Geometry: final body of the model. Coordinates: model frame, mm. Face numbers are marked on the shaded views. A direction names the side the tool comes from. Round coordinates to 2 decimals unless told otherwise and drop trailing zeros. Order: outer loops, then holes, each group sorted by start corner. A loop starts at its lowest first (then second) coordinate and runs counter-clockwise, first axis right, second up. Notation, with made-up numbers: (38.25, -2.5) -> (89.25, -2.5) arc R33 cw to (89.25, 34.5) -> close; hole circle Ø11 at (-28.5, 5.25). An arc over 180 degrees is marked (long way). Put each result on its own line as item: value.
```python
from build123d import *

# Parameters (mm, degrees)
SKETCH10_R           = 4.05
BOSS_EXTRUDE12_DEPTH = 10
SKETCH11_R           = 35
BOSS_EXTRUDE13_DEPTH = 40.8
SKETCH12_R           = 4
BOSS_EXTRUDE14_DEPTH = 6
SKETCH13_R           = 19.993
BOSS_EXTRUDE15_DEPTH = 75
SKETCH16_R           = 39
BOSS_EXTRUDE16_DEPTH = 3
CHAMFER1_SIZE        = 1
CUT_EXTRUDE2_DEPTH   = 131.8


with BuildPart() as part:
    # Sketch10 → Boss-Extrude12 (new body)
    with BuildSketch(Plane(origin=(0, 0, 0), x_dir=(0, 0, -1), z_dir=(1, 0, 0))):
        with BuildLine():
            Line((-55.858638544, -18.55), (-11.864548032, 57.65))
            ThreePointArc((-11.864548032, 57.65), (0, 64.5), (11.864548032, 57.65))
            Line((11.864548032, 57.65), (55.858638544, -18.55))
            ThreePointArc((55.858638544, -18.55), (55.858638544, -32.25), (43.994090512, -39.1))
            Line((43.994090512, -39.1), (-43.994090512, -39.1))
            ThreePointArc((-43.994090512, -39.1), (-55.858638544, -32.25), (-55.858638544, -18.55))
        make_face()
        with Locations((0, 50)):
            Circle(SKETCH10_R, mode=Mode.SUBTRACT)
        with Locations((43.301270189, -25)):
            Circle(SKETCH10_R, mode=Mode.SUBTRACT)
        with Locations((-43.301270189, -25)):
            Circle(SKETCH10_R, mode=Mode.SUBTRACT)
    extrude(amount=BOSS_EXTRUDE12_DEPTH)

    # Sketch11 → Boss-Extrude13 (add)
    with BuildSketch(Plane(origin=(10, 0, 0), x_dir=(0, 0, -1), z_dir=(1, 0, 0))):
        Circle(SKETCH11_R)
    extrude(amount=BOSS_EXTRUDE13_DEPTH)

    # Sketch12 → Boss-Extrude14 (add)
    with BuildSketch(Plane(origin=(50.8, 0, 0), x_dir=(0, 0, -1), z_dir=(1, 0, 0))):
        with BuildLine():
            Line((-43.301270189, 38.7), (43.301270189, 38.7))
            ThreePointArc((43.301270189, 38.7), (55.165818221, 31.85), (55.165818221, 18.15))
            Line((55.165818221, 18.15), (11.864548032, -56.85))
            ThreePointArc((11.864548032, -56.85), (0, -63.7), (-11.864548032, -56.85))
            Line((-11.864548032, -56.85), (-55.165818221, 18.15))
            ThreePointArc((-55.165818221, 18.15), (-55.165818221, 31.85), (-43.301270189, 38.7))
        make_face()
        with Locations((43.301270189, 25)):
            Circle(SKETCH12_R, mode=Mode.SUBTRACT)
        with Locations((0, -50.8)):
            Circle(SKETCH12_R, mode=Mode.SUBTRACT)
        with Locations((-43.301270189, 25)):
            Circle(SKETCH12_R, mode=Mode.SUBTRACT)
    extrude(amount=BOSS_EXTRUDE14_DEPTH)

    # Sketch13 → Boss-Extrude15 (add)
    with BuildSketch(Plane(origin=(56.8, 0, 0), x_dir=(0, 0, -1), z_dir=(1, 0, 0))):
        Circle(SKETCH13_R)
    extrude(amount=BOSS_EXTRUDE15_DEPTH)

    # Sketch16 → Boss-Extrude16 (add)
    with BuildSketch(Plane(origin=(56.8, 0, 0), x_dir=(0, 0, -1), z_dir=(1, 0, 0))):
        with Locations(Location((0, 0, 0), (0, 0, 202.888769737))):
            Circle(SKETCH16_R)
    extrude(amount=BOSS_EXTRUDE16_DEPTH)

    # Chamfer1
    chamfer1_edges = [part.edges().sort_by_distance(p)[0] for p in [
        (131.8, 0, 19.993),
    ]]
    chamfer(chamfer1_edges, length=CHAMFER1_SIZE)

    # Sketch14 → Cut-Extrude2 (cut)
    with BuildSketch(Plane(origin=(131.8, 0, 0), x_dir=(0, 0, -1), z_dir=(1, 0, 0))):
        Polygon((-11.46619671, -6.10543471), (-0.445636795, -12.982734991), (11.020559915, -6.877300281), (11.46619671, 6.10543471), (0.445636795, 12.982734991), (-11.020559915, 6.877300281), align=None)
    extrude(amount=-CUT_EXTRUDE2_DEPTH, mode=Mode.SUBTRACT)


solid = part.part
```
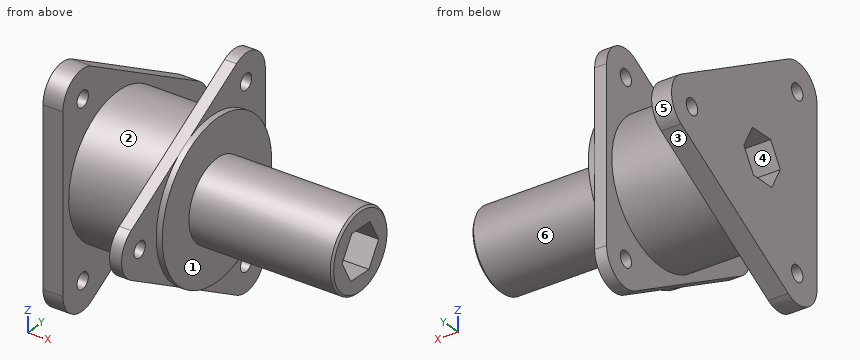
1. Material intervals for probe 1 along Y at (x, z) = (7.75, 0); probe 2 along X at (y, z) = (13.5, -34); probe 3 along X at (y, z) = (-44, -8.5), sorted ascending.
Ans:
probe 1: -39.1 to -12.75, 12.75 to 45.95, 54.05 to 64.5
probe 2: 0 to 10, 50.8 to 59.8
probe 3: 50.8 to 56.8
2. Set-up query: the marked faces 1, 2 and 3. Return all of +Z, -Z, +X, -X, +Y, -Y with unobstructed straight access to the full face (end or side cutting, diameter ignored); none if empty.
Ans:
face 1: +X
face 2: none
face 3: -Z, -X, +Y
3. Cut plane D-D on x = 91.5. Return loops of the section in (y, z), and give its area (3 significant figures).
Ans:
outline: circle Ø39.99 at (0, 0); hole (-12.98, 0.45) -> (-6.88, -11.02) -> (6.11, -11.47) -> (12.98, -0.45) -> (6.88, 11.02) -> (-6.11, 11.47) -> close
area: 817 mm²
4. Draft query along Y for the marked faces 4, 5 and 6. Return one class per face: +Y half, -Y half, draft (parallel to the pull), parting line (faces both ways), or undercut.
Ans:
face 4: undercut
face 5: +Y half
face 6: parting line
5. Cut plane C-C on y = -50.8. Return loops of the section in (x, z).
Ans:
outline: (50.8, -15.36) -> (56.8, -15.36) -> (56.8, -4) -> (50.8, -4) -> close; (50.8, 4) -> (56.8, 4) -> (56.8, 15.36) -> (50.8, 15.36) -> close
6. Cut plane A-A on x = 36. Return loops of the section in (y, z).
Ans:
outline: circle Ø70 at (0, 0); hole (-12.98, 0.45) -> (-6.88, -11.02) -> (6.11, -11.47) -> (12.98, -0.45) -> (6.88, 11.02) -> (-6.11, 11.47) -> close
7. Contact query for flat-ended pins moving along their axis: P1, Ø5.5, axis at y = -18, z = 34, coming from the -X side; P2, Ø15.5, axis at y = 22, z = -38, coming from the +X side; P3, Ø7.5, axis at y = -25, z = -43.3, coming from the -X side; P4, Ø8, axis at x = 4, z = 1, coming from the -Y side. Output: stop coordinate, or through.
Ans:
P1: x = 0
P2: x = 59.8
P3: through
P4: y = -39.1
8. Cut plane B-B on y = 25. Return loops of the section in (x, z).
Ans:
outline: (0, -30.72) -> (10, -30.72) -> (10, -24.49) -> (50.8, -24.49) -> (50.8, -39.3) -> (56.8, -39.3) -> (56.8, -29.93) -> (59.8, -29.93) -> (59.8, 29.93) -> (56.8, 29.93) -> (56.8, 39.3) -> (50.8, 39.3) -> (50.8, 24.49) -> (10, 24.49) -> (10, 30.72) -> (0, 30.72) -> close; (50.8, -57) -> (56.8, -57) -> (56.8, -47.3) -> (50.8, -47.3) -> close; (50.8, 47.3) -> (56.8, 47.3) -> (56.8, 57) -> (50.8, 57) -> close
